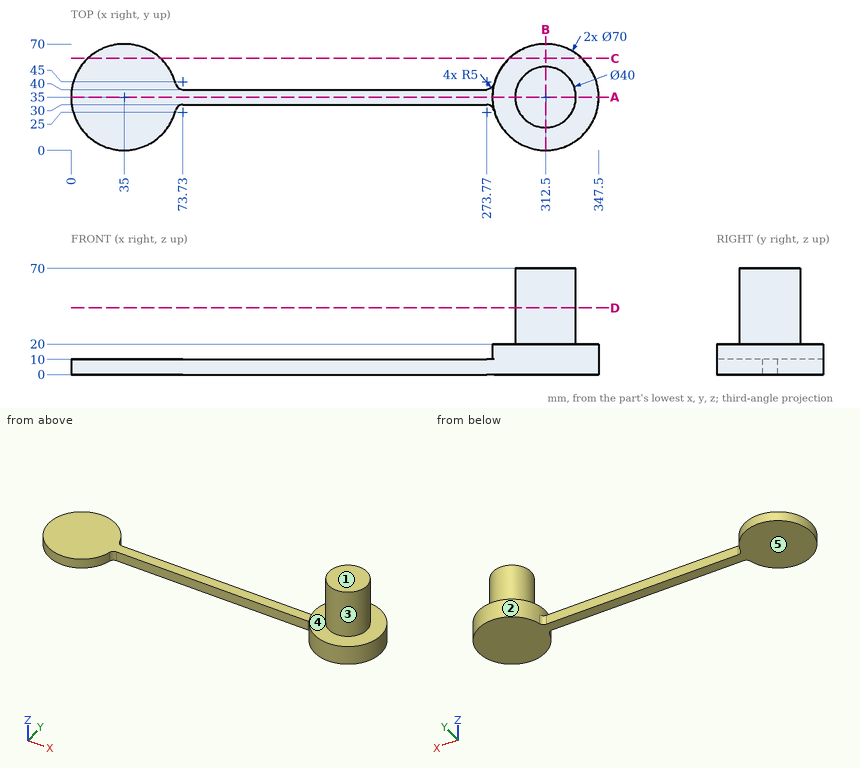
Study the drawing (mm; zero at the part's minimum x, y, z) and answer. A direction names the side the tool comes from. Coordinates: 2 decimals unless noted, no trailing zeros. Write each loop counter-clockwise with the first axis right and the second up, starting at its lowest first coordinate (ties: lowest second). Pieces come first, ordered by that corner, then holes. Notation, with made-up numbers: (27, 40.25) - (56, 40.25) arc R14 ccw to (56, 54.25) - close; hole circle Ø2 at (-8.75, -6.75). An arc over 180 degrees is marked (long way). Answer as a JSON object with one key per item and string values.
Q1. Consider L1, parallel to Z at x = 34, y = 15.5; L2, parallel to Y at x = 300.5, z = 51; L3, parallel to X at y = 42.5, z = 35.5. Determine where each line is inside the solid, lowest interval first. Write a range as from..to.
Results list:
{"L1": "z = 0..10", "L2": "y = 19..51", "L3": "x = 293.96..331.04"}
Q2. For a pull along X with two mould halves and no side action, classify the marked faces 1, 2 and 3 as pulls with the +X half, pulls with the -X half, needs draft (parallel to the pull), parting line crosses it, or undercut.
Results list:
{"face 1": "needs draft", "face 2": "undercut", "face 3": "parting line crosses it"}
Q3. Find section D-D (z = 44). Write down the section's boundary in (x, y).
Results list:
{"outline": "circle Ø40 at (312.5, 35)"}
Q4. Given pin 1 Ø6 at (y, z) = (40.5, 12.5) entering from +X; pin 2 Ø12 at (y, z) = (7, 48.5) entering from +X; pin 3 Ø5 at (y, z) = (49.5, 45.5) entering from -X; pin 4 Ø4 at (x, y) = (46, 40.5) entering from +Z, each flat-ended and moving along its own axis, determine where each tip first touches the part or whether it passes through.
Results list:
{"pin 1": "stops at x = 347.41", "pin 2": "passes through", "pin 3": "stops at x = 296.5", "pin 4": "stops at z = 10"}
Q5. Find section A-A (y = 35). Write down the section's boundary in (x, z), plus the area to 4 significant figures.
Results list:
{"outline": "(0, 0) - (347.5, 0) - (347.5, 20) - (332.5, 20) - (332.5, 70) - (292.5, 70) - (292.5, 20) - (277.5, 20) - (277.5, 10) - (0, 10) - close", "area": "6,175 mm^2"}
Q6. Find section B-B (x = 312.5). Write down the section's boundary in (y, z), plus the area to 3 significant figures.
Results list:
{"outline": "(0, 0) - (70, 0) - (70, 20) - (55, 20) - (55, 70) - (15, 70) - (15, 20) - (0, 20) - close", "area": "3,400 mm^2"}
Q7. Which of the six approach directions +Z, -Z, +X, -X, +Y, -Y give full straight-line access (tool end or side, diameter ignored) to the marked faces 4 and 5?
Results list:
{"face 4": "+Z", "face 5": "-Z, +X, -X, +Y, -Y"}
Q8. Find section C-C (y = 60.5). Write down the section's boundary in (x, z), plus the area to 3 significant figures.
Results list:
{"outline": "(11.03, 0) - (58.97, 0) - (58.97, 10) - (11.03, 10) - close; (288.53, 0) - (336.47, 0) - (336.47, 20) - (288.53, 20) - close", "area": "1,440 mm^2"}
